Design review of the part shown in the three views and the two pictorial views. Dimensions are in mm from the part's minimum x, y and z. A direction names the side the tool comes from. Give positions to 0.01 mm unless a question says otherwise; leave off trailing zeros. Loops run counter-clockwise (first coordinate to the right, second up) from the corner with the lowest first, then second, coordinate; pieces in that order, holes last. Notation, with made-up numbers: (66, -17) -> (87, -17) arc R16 ccw to (87, 3) -> close; hole circle Ø1 at (85.5, 79). An arc over 180 degrees is marked (long way). Answer as CSV lines item,"result".
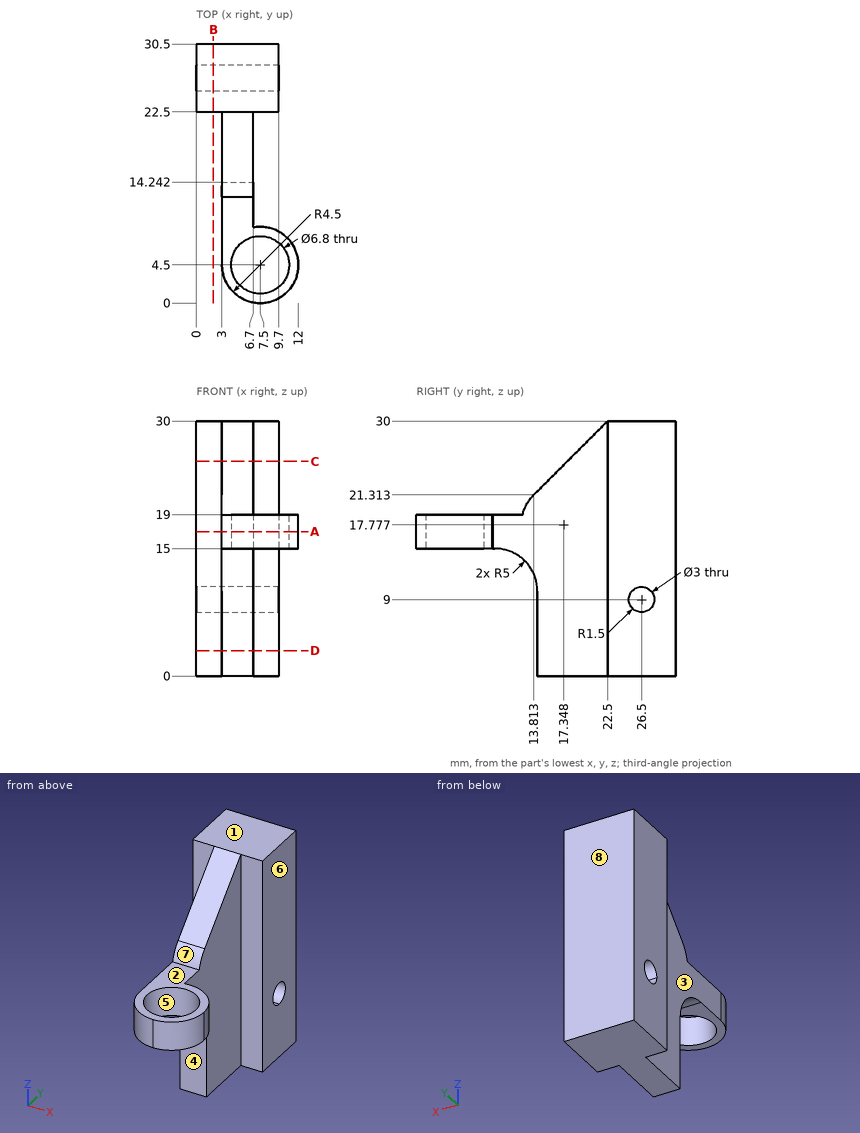
Q1. For the marked faces 1, 2, 3 and 4, list the 3-axis set-ups (+Z, -Z, +X, -X, +Y, -Y) from which the entire face can be reached by the end or side of a thin tool; tool diameter is ignored.
Filled sheet:
face 1,"+Z, +X, -X, +Y, -Y"
face 2,"+Z, +X, -X, -Y"
face 3,"+Z, -Z, -X, -Y"
face 4,"-Z, +X, -X, -Y"
Q2. To check wall thickness, follow probe 1 along Y at (x, z) = (7.5, 17.45); probe 2 along X at (y, z) = (4.5, 18.15); probe 3 along Z at (x, y) = (7.75, 26.5). State the ranges of each line that lie inside material, in increasing order. Write a range as from..to.
Filled sheet:
probe 1,"y = 0..1.1, 7.9..9, 22.5..30.5"
probe 2,"x = 3..4.1, 10.9..12"
probe 3,"z = 0..7.5, 10.5..30"
Q3. The part is to be moulded in two halves that separate along Y. For the marked faces 5, 6, 7 and 8, say which applies: pulls with the +Y half, pulls with the -Y half, needs draft (parallel to the pull), parting line crosses it, or undercut.
Filled sheet:
face 5,"undercut"
face 6,"needs draft"
face 7,"pulls with the -Y half"
face 8,"pulls with the +Y half"
Q4. We need section C-C, the plane z = 25.25. State the section outline as (x, y) points.
Filled sheet:
outline,"(0, 22.5) -> (3, 22.5) -> (3, 17.75) -> (6.7, 17.75) -> (6.7, 22.5) -> (9.7, 22.5) -> (9.7, 30.5) -> (0, 30.5) -> close"
Q5. We need section D-D, the plane z = 3. State the section outline as (x, y) points.
Filled sheet:
outline,"(0, 22.5) -> (3, 22.5) -> (3, 14.24) -> (6.7, 14.24) -> (6.7, 22.5) -> (9.7, 22.5) -> (9.7, 30.5) -> (0, 30.5) -> close"
Q6. We need section A-A, the plane z = 17. State the section outline as (x, y) points.
Filled sheet:
outline,"(0, 22.5) -> (3, 22.5) -> (3, 4.5) arc R4.5 ccw (long way) to (6.7, 8.93) -> (6.7, 22.5) -> (9.7, 22.5) -> (9.7, 30.5) -> (0, 30.5) -> close; hole circle Ø6.8 at (7.5, 4.5)"
Q7. Clearance check with flat-ended pins moving along their axes: pin 1 Ø4 at (y, z) = (16.5, 13) entering from +X; pin 2 Ø6 at (x, y) = (7.5, 4.5) entering from -Z; pin 3 Ø9 at (y, z) = (28, 15.5) entering from +X; pin 4 Ø3.5 at (x, z) = (2, 15.5) entering from -Y. State where each tip first meets the part, or that it passes through.
Filled sheet:
pin 1,"stops at x = 6.7"
pin 2,"passes through"
pin 3,"stops at x = 9.7"
pin 4,"stops at y = 2.01"
Q8. We need section B-B, the plane x = 2. State the section outline as (y, z) points, and give its area (3 significant figures).
Filled sheet:
outline,"(22.5, 0) -> (30.5, 0) -> (30.5, 30) -> (22.5, 30) -> close; hole circle Ø3 at (26.5, 9)"
area,"233 mm^2"
